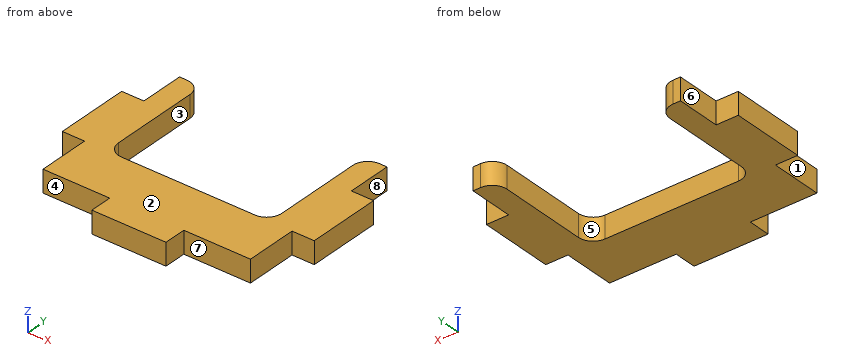
from build123d import *

# Parameters (mm, degrees)
SKETCH_1_W               = 28
SKETCH_1_H               = 24
SKETCH_1_W_2             = 3
SKETCH_1_H_2             = 10
SKETCH_1_W_3             = 10
SKETCH_1_H_3             = 3
EXTRUDE_1_DEPTH          = 3
SKETCH_3_W               = 28
SKETCH_3_H               = 1
CUT_EXTRUDE_2_DEPTH      = 3
CUT_EXTRUDE_3_DEPTH      = 23.869193252
CUT_EXTRUDE_3_DEPTH_BACK = 23.869193252
SKETCH_4_W               = 22
SKETCH_4_H               = 16
FILLET_1_R               = 2


with BuildPart() as part:
    # 草图1 → 凸台-拉伸1 (new body)
    with BuildSketch(Plane.XY):
        Rectangle(SKETCH_1_W, SKETCH_1_H)
        with Locations((-15.5, 0)):
            Rectangle(SKETCH_1_W_2, SKETCH_1_H_2)
        with Locations((15.5, 0)):
            Rectangle(SKETCH_1_W_2, SKETCH_1_H_2)
        with Locations((0, -13.5)):
            Rectangle(SKETCH_1_W_3, SKETCH_1_H_3)
    extrude(amount=EXTRUDE_1_DEPTH)

    # 草图3 → 切除-拉伸2 (cut)
    with BuildSketch(Plane.XY.offset(3)):
        with Locations((0, 11.5)):
            Rectangle(SKETCH_3_W, SKETCH_3_H)
    extrude(amount=-CUT_EXTRUDE_2_DEPTH, mode=Mode.SUBTRACT)

    # 草图4 → 切除-拉伸3 (cut, two sides: drawn at the far end of the back side and taken through both)
    with BuildSketch(Plane.XY.offset(3).offset(-CUT_EXTRUDE_3_DEPTH_BACK)):
        with Locations((0, 3)):
            Rectangle(SKETCH_4_W, SKETCH_4_H)
    extrude(amount=CUT_EXTRUDE_3_DEPTH + CUT_EXTRUDE_3_DEPTH_BACK, mode=Mode.SUBTRACT)

    # 圆角1
    fillet_1_edges = [part.edges().sort_by_distance(p)[0] for p in [
        (-11, -5, 1.5),
        (-11, 11, 1.5),
        (11, 11, 1.5),
        (11, -5, 1.5),
    ]]
    fillet(fillet_1_edges, radius=FILLET_1_R)


solid = part.part
Can you work these out from the model? Positions are in its coordinate system, mm. Face numbers are marked on the shaded views. A direction names the side the tool comes from. Give positions to 0.01 mm unless a question says otherwise; leave off trailing zeros. Loops run counter-clockwise (first coordinate to the right, second up) from the corner with the lowest first, then second, coordinate; pieces in that order, holes last. Notation, with made-up numbers: M 4.25,10.5 L 63.25,10.5 A23 ccw 63.25,39.5 Z; hole C -3,44.25 d8. An arc over 180 degrees is marked long. One line per item, written item: value. Start each with the question number.
1) If I drill on line 1 (X direction, y = 4.25, z = 0.9); line 2 (X direction, y = 6.5, z = 2.05); line 3 (X direction, y = -13.5, z = 1.6), over which ranges is the centre line in solid material (lowest first)? Write a range as [from, to].
2) I'm going to push flat-ended pins straight in: pin 1 (2 mm diameter, centred on x = 13, y = -4.5, fed in from -Z); pin 2 (1 mm diameter, centred on x = 6.5, z = 1.5, fed in from -Y); pin 3 (1.5 mm diameter, centred on y = 6.5, z = 1.5, fed in from +X); pin 4 (0.9 mm diameter, centred on y = -9, z = 2, fed in from -X). Where does each tip first touch, or does it pass through?
3) If we section it at B-B, the plane z = 1.1: Write out the boundary of the cut face in (x, y), and give its area (3 significant figures).
4) If we section it at D-D, the plane y = -7: Write out the boundary of the cut face in (x, z).
5) On a 3-axis mill with a long thin cutter (end or side, diameter ignored), from which of +Z, -Z, +X, -X, +Y, -Y can I reach the whole of each face in a straight line? I mean the marked faces 4, 5, 6, 7 and 8. Say none if no direction works.
6) If we section it at C-C, the plane y = 6.5: Write out the boundary of the cut face in (x, z).
7) Thinking about a two-plate mould opening in X: for the marked faces 1, 2 and 3, which applies, +X half, -X half, draft (parallel to the pull), parting line (faces both ways), or undercut?
8) If we section it at A-A, the plane y = 1.5: Write out the boundary of the cut face in (x, z).
Completed:
1. line 1: x = [-17, -11], [11, 17]
1. line 2: x = [-14, -11], [11, 14]
1. line 3: x = [-5, 5]
2. pin 1: stops at z = 0
2. pin 2: stops at y = -12
2. pin 3: stops at x = 14
2. pin 4: stops at x = -14
3. outline: M -17,-5 L -14,-5 L -14,-12 L -5,-12 L -5,-15 L 5,-15 L 5,-12 L 14,-12 L 14,-5 L 17,-5 L 17,5 L 14,5 L 14,11 L 13,11 A2 ccw 11,9 L 11,-3 A2 cw 9,-5 L -9,-5 A2 cw -11,-3 L -11,9 A2 ccw -13,11 L -14,11 L -14,5 L -17,5 Z
3. area: 382 mm^2
4. outline: M -14,0 L 14,0 L 14,3 L -14,3 Z
5. face 4: +Z, -Z, -X, -Y
5. face 5: +Z, -Z, +Y
5. face 6: +Z, -Z, -X, +Y
5. face 7: +Z, -Z, +X, -Y
5. face 8: +Z, -Z, +X, +Y
6. outline: M -14,0 L -11,0 L -11,3 L -14,3 Z; M 11,0 L 14,0 L 14,3 L 11,3 Z
7. face 1: -X half
7. face 2: draft
7. face 3: undercut
8. outline: M -17,0 L -11,0 L -11,3 L -17,3 Z; M 11,0 L 17,0 L 17,3 L 11,3 Z
